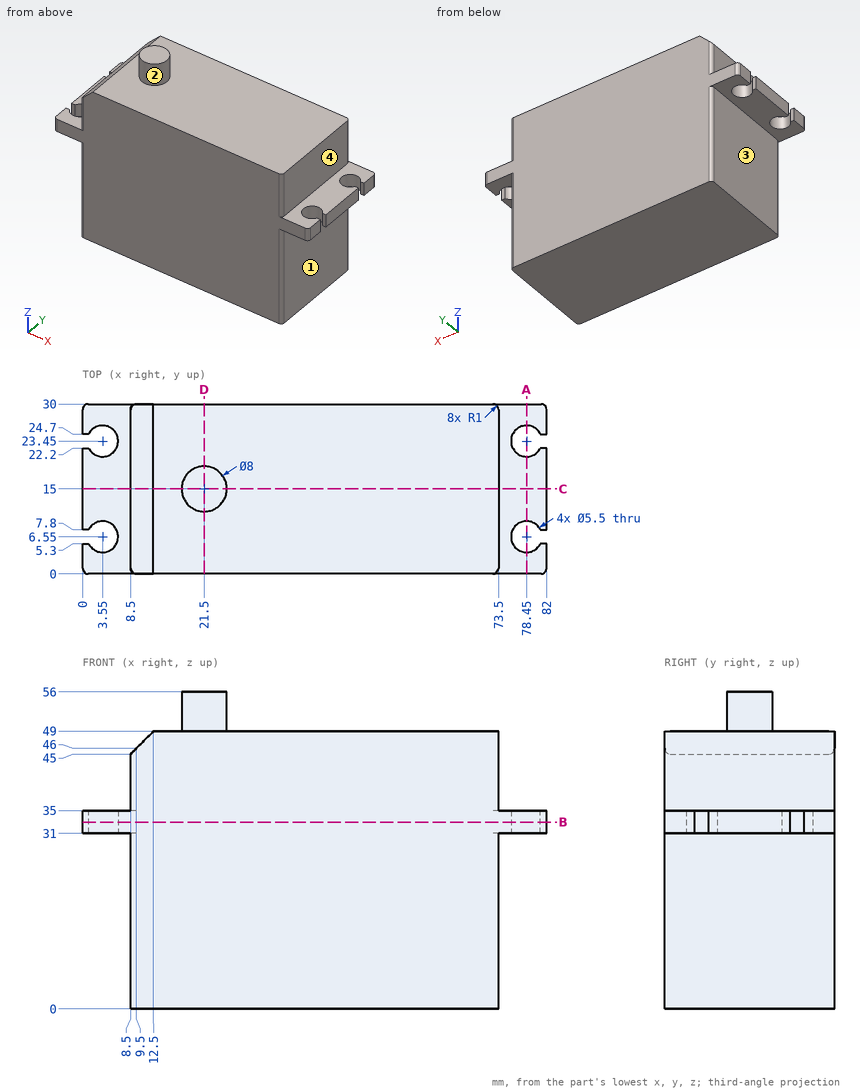
Study the drawing (mm; zero at the part's minimum x, y, z) and answer. A direction names the side the tool comes from. Give positions to 0.01 mm unless a question says otherwise; leave off trailing zeros. Write each loop counter-clockwise with the first axis right and the second up, starting at its lowest first coordinate (ties: lowest second). Pieces come first, ordered by that corner, then holes. Notation, with made-up numbers: (28, 46.5) -> (57, 46.5) arc R12 ccw to (57, 50.5) -> close; hole circle Ø2 at (-9.5, 22.5). An arc over 180 degrees is marked (long way). Write item = value, one per line. Start each with the question number.
1) Each of these flat-tipped pins is pushed along its axis until it touches: pin 1 (8.5 mm diameter, centred on y = 12.5, z = 8, fed in from -X); pin 2 (10.5 mm diameter, centred on x = 78, y = 14.5, fed in from +Z); pin 3 (6.5 mm diameter, centred on x = 78.45, y = 23.45, fed in from -Z). Where does it stop, or does it pass through?
2) The part is cut by section C-C, the plane y = 15. Determine the outline of the cut face in (x, z).
3) The part is cut by section D-D, the plane x = 21.5. Determine the outline of the cut face in (y, z), and give its area (3 significant figures).
4) The part is cut by section B-B, the plane z = 33. Determine the outline of the cut face in (x, y).
5) Straight lines are drawn through the part: line 1 along Y through (x, z) = (78.45, 32.9); line 2 along Z through (x, y) = (48.5, 1.5); line 3 along X through (y, z) = (23.75, 43). For each, find the intervals that lie inside material, in ascending order.
6) The part is cut by section A-A, the plane x = 78.45. Determine the outline of the cut face in (y, z), and give its area (3 significant figures).
7) Which of the six approach directions +Z, -Z, +X, -X, +Y, -Y give full straight-line access (tool end or side, diameter ignored) to the marked faces 1, 2, 3 and 4?
Solutions:
q1.pin_1 = 8.5
q1.pin_2 = 49
q1.pin_3 = 31
q2.outline = (0, 31) -> (8.5, 31) -> (8.5, 0) -> (73.5, 0) -> (73.5, 31) -> (82, 31) -> (82, 35) -> (73.5, 35) -> (73.5, 49) -> (25.5, 49) -> (25.5, 56) -> (17.5, 56) -> (17.5, 49) -> (12.5, 49) -> (8.5, 45) -> (8.5, 35) -> (0, 35) -> close
q3.outline = (0, 0) -> (30, 0) -> (30, 49) -> (19, 49) -> (19, 56) -> (11, 56) -> (11, 49) -> (0, 49) -> close
q3.area = 1,530 mm²
q4.outline = (0, 1) arc R1 ccw to (1, 0) -> (81, 0) arc R1 ccw to (82, 1) -> (82, 5.3) -> (80.9, 5.3) arc R2.75 cw (long way) to (80.9, 7.8) -> (82, 7.8) -> (82, 22.2) -> (80.9, 22.2) arc R2.75 cw (long way) to (80.9, 24.7) -> (82, 24.7) -> (82, 29) arc R1 ccw to (81, 30) -> (1, 30) arc R1 ccw to (0, 29) -> (0, 24.7) -> (1.1, 24.7) arc R2.75 cw (long way) to (1.1, 22.2) -> (0, 22.2) -> (0, 7.8) -> (1.1, 7.8) arc R2.75 cw (long way) to (1.1, 5.3) -> (0, 5.3) -> close
q5.line_1 = 0 to 3.8, 9.3 to 20.7, 26.2 to 30
q5.line_2 = 0 to 49
q5.line_3 = 8.5 to 73.5
q6.outline = (0, 31) -> (3.8, 31) -> (3.8, 35) -> (0, 35) -> close; (9.3, 31) -> (20.7, 31) -> (20.7, 35) -> (9.3, 35) -> close; (26.2, 31) -> (30, 31) -> (30, 35) -> (26.2, 35) -> close
q6.area = 76.0 mm²
q7.face_1 = -Z, +X, +Y, -Y
q7.face_2 = +Z
q7.face_3 = -Z, -X, +Y, -Y
q7.face_4 = +Z, +X, +Y, -Y
